The drawing under review shows one solid part. Ordinate dimensions are in mm from its lowest x, y, z. A direction names the side the tool comes from. Coordinates: 2 decimals unless noted, no trailing zeros. Write each loop counter-clockwise with the first axis right and the second up, starting at its lowest first coordinate (ties: lowest second). Pieces come first, ordered by that corner, then holes.
1) For P1, Ø1, axis at x = 31, y = 9.5, coming from the +Z side; P2, Ø1.5, axis at y = 4.5, z = 7, coming from the -X side; P3, Ø2.5, axis at x = 33.76, y = 5.72, coming from the +Z side; P4, Ø6, axis at y = 9.5, z = 11, coming from the +X side, all flat-tipped, find the tip position at first contact; note any pin that passes through.
2) Add section C-C, the plane y = 9.5. State the section outline as (x, z) points.
3) Mouldability with a two-part tool opening along X and no side actions: class the marked faces 1, 2, 3 and 4 as released by +X, released by -X, zero draft, split by the parting line, or undercut.
4) Add section A-A, the plane z = 5. State the section outline as (x, y) points.
5) Machinability: for the marked faces 5, 6, 7, 8 and 9, which of the approach directions +Z, -Z, +X, -X, +Y, -Y give a long, thin tool a straight path to every point of the face, cutting with its end or side? Answer none if there is none.
6) Add section B-B, the plane x = 33. State the section outline as (y, z) points (1 decimal).
7) Add section D-D, the plane z = 1.5. State the section outline as (x, y) points (1 decimal), then the cut area to 3 significant figures.
8) For line 1 (X direction, y = 1.5, z = 3.75); line 2 (X direction, y = 5.5, z = 9); line 3 (Y direction, x = 6, z = 3), list the stretches that pass through material, from the lowest coordinate up.
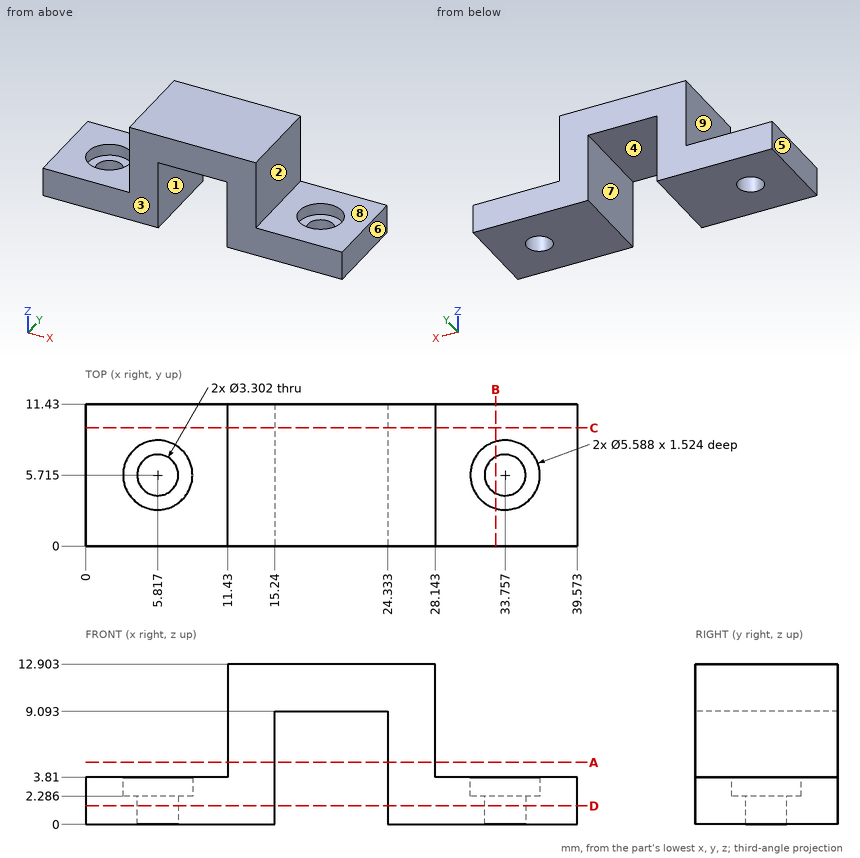
Geometry results:
1. P1: stops at z = 3.81
1. P2: stops at x = 11.43
1. P3: passes through
1. P4: stops at x = 28.14
2. outline: (0, 0) - (15.24, 0) - (15.24, 9.09) - (24.33, 9.09) - (24.33, 0) - (39.57, 0) - (39.57, 3.81) - (28.14, 3.81) - (28.14, 12.9) - (11.43, 12.9) - (11.43, 3.81) - (0, 3.81) - close
3. face 1: undercut
3. face 2: released by +X
3. face 3: zero draft
3. face 4: undercut
4. outline: (11.43, 0) - (15.24, 0) - (15.24, 11.43) - (11.43, 11.43) - close; (24.33, 0) - (28.14, 0) - (28.14, 11.43) - (24.33, 11.43) - close
5. face 5: +Z, -Z, -X, +Y, -Y
5. face 6: +Z, -Z, +X, +Y, -Y
5. face 7: -Z, +Y, -Y
5. face 8: +Z, +X, +Y, -Y
5. face 9: +Z, -X, +Y, -Y
6. outline: (0, 0) - (4.2, 0) - (4.2, 2.3) - (3, 2.3) - (3, 3.8) - (0, 3.8) - close; (7.2, 0) - (11.4, 0) - (11.4, 3.8) - (8.4, 3.8) - (8.4, 2.3) - (7.2, 2.3) - close
7. outline: (0, 0) - (15.2, 0) - (15.2, 11.4) - (0, 11.4) - close; (24.3, 0) - (39.6, 0) - (39.6, 11.4) - (24.3, 11.4) - close; hole circle Ø3.3 at (5.8, 5.7); hole circle Ø3.3 at (33.8, 5.7)
7. area: 331 mm2
8. line 1: x = 0 to 15.24, 24.33 to 39.57
8. line 2: x = 11.43 to 15.24, 24.33 to 28.14
8. line 3: y = 0 to 2.93, 8.5 to 11.43
